Could you check a few things on this model? Use its own coordinates, in mm. A direction names the side the tool comes from. Round coordinates to 2 decimals unless told otherwise and drop trailing zeros. Write each loop counter-clockwise with the first axis right and the second up, starting at its lowest first coordinate (ties: lowest second). Pieces come first, ordered by that corner, then holes. Notation, with made-up numbers: (-23, 82.25) - (3, 82.25) arc R37 cw to (3, 121.25) - close; hole circle Ø5 at (9, 74). An arc over 180 degrees is marked (long way). Write each question's results on one line, items separated by ' | '. Start each with the question number.
(1) Imagine slicing it at A-A on z = 3.5. Write out the boundary of the cut face in (x, y), then the cut area to 3 significant figures.
(2) Imagine slicing it at B-B on x = -4.5. Write out the boundary of the cut face in (y, z), then the cut area to 3 significant figures.
(3) Imagine slicing it at C-C on y = 3. Write out the boundary of the cut face in (x, z).
(4) Imagine slicing it at D-D on x = 13. Write out the boundary of the cut face in (y, z), then the cut area to 3 significant figures.
(5) For P1, Ø8, axis at x = 6, y = -8, coming from the +Z side; P2, Ø1.6, axis at x = -20.5, y = -9, coming from the +Z side; P3, Ø5, axis at x = 12, z = 6, coming from the +Y side, each with a flat end and sliding along its axis, tell me the tip position at first contact or that it passes through.
(6) Thinking about a two-plate mould opening in X: for faces 1 (the flat face through (4, 0, 1.7)), 2 (the cylindrical face through (1.265, 4.549, 5.249)), 3 (the flat face through (20, -9, -0.1)), 4 (the cylindrical face through (-10.149, -6.865, 5.249)), which applies, +X half, -X half, draft (parallel to the pull), parting line (faces both ways), or undercut?
(7) Please list where these lines run through material, in increasing order: line 1 (Y direction, x = -11, z = 0.85); line 2 (X direction, y = 8.15, z = 0.95); line 3 (X direction, y = -8.15, z = 1.05). Write a range as [from, to].
(8) On a 3-axis mill with a long thin cutter (end or side, diameter ignored), from which of +Z, -Z, +X, -X, +Y, -Y can I reach the whole of each face in a straight line? I mean faces 5 (the flat face through (-5, 4.85, 5)), 6 (the flat face through (-20, -9, 1.8)), 7 (the cylindrical face through (1.249, -6.865, 5.249)), 8 (the flat face through (-5, -1, 8.7)). Say none if no direction works.
```python
from build123d import *

# Parameters (mm, degrees)
SKETCH1_W           = 42
SKETCH1_H           = 20.3
BOSS_EXTRUDE1_DEPTH = 1.7
BOSS_EXTRUDE2_START = 1.7
SKETCH1_3_R         = 5
BOSS_EXTRUDE2_DEPTH = 11
BOSS_EXTRUDE3_START = 1.7
SKETCH1_4_W         = 12
SKETCH1_4_H         = 12
BOSS_EXTRUDE3_DEPTH = 7
FILLET1_R           = 1
SKETCH1_5_R         = 1.5
CUT_EXTRUDE1_DEPTH  = 27.557720158
BOSS_EXTRUDE4_START = -0.1
SKETCH1_6_W         = 2
SKETCH1_6_H         = 2
BOSS_EXTRUDE4_DEPTH = 1.9


with BuildPart() as part:
    # Sketch1 → Boss-Extrude1 (new body)
    with BuildSketch(Plane.XY):
        Rectangle(SKETCH1_W, SKETCH1_H)
    extrude(amount=BOSS_EXTRUDE1_DEPTH)

    # Sketch1<3> → Boss-Extrude2 (add)
    with BuildSketch(Plane.XY.offset(BOSS_EXTRUDE2_START)):
        with Locations((-15.95, 0)):
            Circle(SKETCH1_3_R)
        with Locations((15.9, 0)):
            Circle(SKETCH1_3_R)
    extrude(amount=BOSS_EXTRUDE2_DEPTH)

    # Sketch1<4> → Boss-Extrude3 (add)
    with BuildSketch(Plane.XY.offset(BOSS_EXTRUDE3_START)):
        with Locations((-4.45, -1.15)):
            Rectangle(SKETCH1_4_W, SKETCH1_4_H)
    extrude(amount=BOSS_EXTRUDE3_DEPTH)

    # Fillet1
    fillet1_edges = [part.edges().sort_by_distance(p)[0] for p in [
        (-10.45, 4.85, 5.2),
        (-10.45, -7.15, 5.2),
        (1.55, -7.15, 5.2),
        (1.55, 4.85, 5.2),
    ]]
    fillet(fillet1_edges, radius=FILLET1_R)

    # Sketch1<5> → Cut-Extrude1 (cut, through all)
    with BuildSketch(Plane.XY):
        with Locations((-11, 8.15)):
            Circle(SKETCH1_5_R)
        with Locations((13, -8.15)):
            Circle(SKETCH1_5_R)
    extrude(amount=CUT_EXTRUDE1_DEPTH, mode=Mode.SUBTRACT)

    # Sketch1<6> → Boss-Extrude4 (add)
    with BuildSketch(Plane.XY.offset(BOSS_EXTRUDE4_START)):
        with Locations((20, 9.15)):
            Rectangle(SKETCH1_6_W, SKETCH1_6_H)
        with Locations((-20, 9.15)):
            Rectangle(SKETCH1_6_W, SKETCH1_6_H)
        with Locations((20, -9.15)):
            Rectangle(SKETCH1_6_W, SKETCH1_6_H)
        with Locations((-20, -9.15)):
            Rectangle(SKETCH1_6_W, SKETCH1_6_H)
    extrude(amount=BOSS_EXTRUDE4_DEPTH)


solid = part.part
```
Response:
1) outline: circle Ø10 at (-15.95, 0); (-10.45, -6.15) arc R1 ccw to (-9.45, -7.15) - (0.55, -7.15) arc R1 ccw to (1.55, -6.15) - (1.55, 3.85) arc R1 ccw to (0.55, 4.85) - (-9.45, 4.85) arc R1 ccw to (-10.45, 3.85) - close; circle Ø10 at (15.9, 0) | area: 300 mm²
2) outline: (-10.15, 0) - (10.15, 0) - (10.15, 1.7) - (4.85, 1.7) - (4.85, 8.7) - (-7.15, 8.7) - (-7.15, 1.7) - (-10.15, 1.7) - close | area: 119 mm²
3) outline: (-21, 0) - (21, 0) - (21, 1.7) - (19.9, 1.7) - (19.9, 12.7) - (11.9, 12.7) - (11.9, 1.7) - (1.55, 1.7) - (1.55, 8.7) - (-10.45, 8.7) - (-10.45, 1.7) - (-11.95, 1.7) - (-11.95, 12.7) - (-19.95, 12.7) - (-19.95, 1.7) - (-21, 1.7) - close
4) outline: (-10.15, 0) - (-9.65, 0) - (-9.65, 1.7) - (-10.15, 1.7) - close; (-6.65, 0) - (10.15, 0) - (10.15, 1.7) - (4.07, 1.7) - (4.07, 12.7) - (-4.07, 12.7) - (-4.07, 1.7) - (-6.65, 1.7) - close | area: 119 mm²
5) P1: z = 1.7 | P2: z = 1.8 | P3: y = 4.8
6) face 1: undercut | face 2: undercut | face 3: draft | face 4: -X half
7) line 1: [-10.15, 6.65], [9.65, 10.15] | line 2: [-21, -12.5], [-9.5, 21] | line 3: [-21, 11.5], [14.5, 21]
8) face 5: +Z, +Y | face 6: +Z, +X, -X, -Y | face 7: +Z, +X, -Y | face 8: +Z, +Y, -Y
